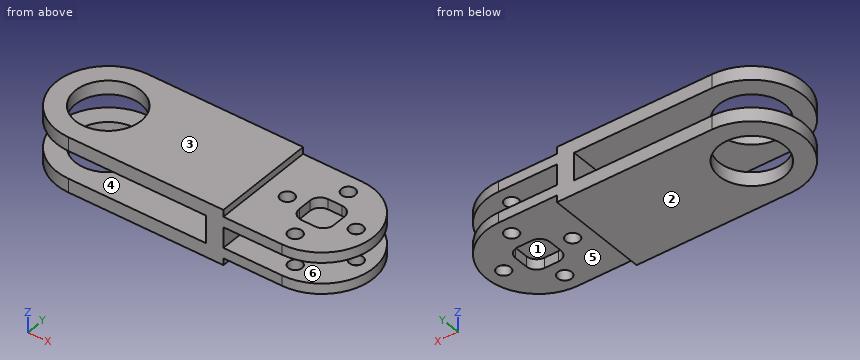
from build123d import *

# Parameters (mm, degrees)
EXTRUDE_1_DEPTH          = 16
SKETCH_2_R               = 9.5
SKETCH_2_R_2             = 2
SKETCH_2_W               = 10
SKETCH_2_H               = 10
CUT_EXTRUDE_1_DEPTH      = 16
FILLET_1_R               = 3
CUT_EXTRUDE_5_DEPTH      = 15
CUT_EXTRUDE_5_DEPTH_BACK = 15
SKETCH_4_W               = 55
SKETCH_4_H               = 8
CUT_EXTRUDE_6_DEPTH      = 15
CUT_EXTRUDE_6_DEPTH_BACK = 15
SKETCH_5_W               = 32
SKETCH_5_H               = 2


with BuildPart() as part:
    # 草图1 → 凸台-拉伸1 (new body)
    with BuildSketch(Plane.XY):
        with BuildLine():
            Line((0, 15), (62, 15))
            ThreePointArc((62, 15), (77, 0), (62, -15))
            Line((62, -15), (0, -15))
            ThreePointArc((0, -15), (-15, 0), (0, 15))
        make_face()
    extrude(amount=EXTRUDE_1_DEPTH)

    # 草图2 → 切除-拉伸1 (cut)
    with BuildSketch(Plane.XY.offset(16)):
        Circle(SKETCH_2_R)
        with Locations((62, 10)):
            Circle(SKETCH_2_R_2)
        with Locations((72, 0)):
            Circle(SKETCH_2_R_2)
        with Locations((62, -10)):
            Circle(SKETCH_2_R_2)
        with Locations((52, 0)):
            Circle(SKETCH_2_R_2)
        with Locations((62, 0)):
            Rectangle(SKETCH_2_W, SKETCH_2_H)
    extrude(amount=-CUT_EXTRUDE_1_DEPTH, mode=Mode.SUBTRACT)

    # 圆角1
    fillet_1_edges = [part.edges().sort_by_distance(p)[0] for p in [
        (67, 5, 8),
        (67, -5, 8),
        (57, -5, 8),
        (57, 5, 8),
    ]]
    fillet(fillet_1_edges, radius=FILLET_1_R)

    # 草图4 → 切除-拉伸5 (cut, two sides: drawn at the far end of the back side and taken through both)
    with BuildSketch(Plane(origin=(0, 0, 0), x_dir=(1, 0, 0), z_dir=(0, 1, 0)).offset(-CUT_EXTRUDE_5_DEPTH_BACK)):
        with Locations((12.5, -8)):
            Rectangle(SKETCH_4_W, SKETCH_4_H)
    extrude(amount=CUT_EXTRUDE_5_DEPTH + CUT_EXTRUDE_5_DEPTH_BACK, mode=Mode.SUBTRACT)

    # 草图5 → 切除-拉伸6 (cut, two sides: drawn at the far end of the back side and taken through both)
    with BuildSketch(Plane(origin=(0, 0, 0), x_dir=(1, 0, 0), z_dir=(0, 1, 0)).offset(-CUT_EXTRUDE_6_DEPTH_BACK)):
        Polygon((45, -8), (45, -11), (77, -11), (77, -5), (45, -5), align=None)
        with Locations((61, -1)):
            Rectangle(SKETCH_5_W, SKETCH_5_H)
        with Locations((61, -15)):
            Rectangle(SKETCH_5_W, SKETCH_5_H)
    extrude(amount=CUT_EXTRUDE_6_DEPTH + CUT_EXTRUDE_6_DEPTH_BACK, mode=Mode.SUBTRACT)


solid = part.part
Could you check a few things on this model? Use its own coordinates, in mm. Face numbers are marked on the shaded views. A direction names the side the tool comes from. Round coordinates to 2 decimals unless told otherwise and drop trailing zeros. Order: outer loops, then holes, each group sorted by start corner. A loop starts at its lowest first (then second) coordinate and runs counter-clockwise, first axis right, second up. Notation, with made-up numbers: M -39.5,-18.75 L 13.5,-18.75 A36 ccw 13.5,15.25 Z; hole C -29,61 d6. An arc over 180 degrees is marked long. One line per item, written item: value.
(1) I need wall thicknesses on line 1 along Y through (x, z) = (62, 13.1); line 2 along Z through (x, y) = (30, 11); line 3 along Y through (x, z) = (52, 3.95). Which ranges of each line are inside material? Lowest first, please. Write a range as from..to.
Ans:
line 1: y = -15..-12, -8..-5, 5..8, 12..15
line 2: z = 0..4, 12..16
line 3: y = -15..-2, 2..15
(2) Imagine slicing it at A-A (x = 18.5). Write out the boundary of the cut face in (y, z), and give its area (3 significant figures).
Ans:
outline: M -15,0 L 15,0 L 15,4 L -15,4 Z; M -15,12 L 15,12 L 15,16 L -15,16 Z
area: 240 mm^2
(3) Imagine slicing it at D-D (y = 0). Count the separate pieces of the cut face and the enclosed holes in it, and give its area (3 significant figures).
Ans:
separate pieces: 9
enclosed holes: 0
area: 452 mm^2
(4) If we mould it in two halves opening along Z, with no side actions, what happens to the marked faces 1, 2 and 3? For each: released by +Z, released by -Z, zero draft, split by the parting line, or undercut.
Ans:
face 1: undercut
face 2: released by -Z
face 3: released by +Z
(5) Imagine slicing it at C-C (y = 11). Write out the boundary of the cut face in (x, z), and give its area (3 significant figures).
Ans:
outline: M -10.2,0 L 45,0 L 45,2 L 60.27,2 L 60.27,5 L 45,5 L 45,11 L 60.27,11 L 60.27,14 L 45,14 L 45,16 L -10.2,16 L -10.2,12 L 40,12 L 40,4 L -10.2,4 Z; M 63.73,2 L 72.2,2 L 72.2,5 L 63.73,5 Z; M 63.73,11 L 72.2,11 L 72.2,14 L 63.73,14 Z
area: 624 mm^2
(6) I'm going to push flat-ended pins straight in: P1, Ø1, axis at y = 1, z = 1, coming from the +X side; P2, Ø6, axis at y = 11.5, z = 11, coming from the +X side; P3, Ø6, axis at x = -5, z = 11, coming from the +Y side. Where does each tip first touch, or does it pass through?
Ans:
P1: stops at x = 45
P2: stops at x = 74.36
P3: stops at y = 14.84
(7) Which directions (+Z, -Z, +X, -X, +Y, -Y) give clear straight access to the entire face, cutting with the end or side of a thin tool? Please do the marked faces 4, 5 and 6.
Ans:
face 4: -X, +Y, -Y
face 5: -Z, +X, +Y, -Y
face 6: +X, +Y, -Y
(8) Imagine slicing it at B-B (x = 52). Write out the boundary of the cut face in (y, z).
Ans:
outline: M -15,2 L -2,2 L -2,5 L -15,5 Z; M -15,11 L -2,11 L -2,14 L -15,14 Z; M 2,2 L 15,2 L 15,5 L 2,5 Z; M 2,11 L 15,11 L 15,14 L 2,14 Z
